```python
from build123d import *

# Parameters (mm, degrees)
SKETCH1_R           = 1.65
BOSS_EXTRUDE1_DEPTH = 30
SKETCH2_R           = 3
BOSS_EXTRUDE2_DEPTH = 3
FILLET1_R           = 5


with BuildPart() as part:
    # Sketch1 → Boss-Extrude1 (new body)
    with BuildSketch(Plane(origin=(0, 0, 0), x_dir=(1, 0, 0), z_dir=(0, 1, 0))):
        with Locations(Location((0, 0, 0), (0, 0, 270))):
            Circle(SKETCH1_R)
    extrude(amount=BOSS_EXTRUDE1_DEPTH)

    # Sketch2 → Boss-Extrude2 (add)
    with BuildSketch(Plane(origin=(0, 30, 0), x_dir=(1, 0, 0), z_dir=(0, 1, 0))):
        with Locations(Location((0, 0, 0), (0, 0, 270))):
            Circle(SKETCH2_R)
    extrude(amount=BOSS_EXTRUDE2_DEPTH)

    # Fillet1
    # the kernel refuses this fillet: 5 mm, written as the material it adds along each edge
    with BuildSketch(Plane(origin=(0, 30, 0), x_dir=(0, 0, 1), z_dir=(-1, 0, 0))) as fillet1_piece_1:
        with BuildLine():
            CenterArc((6.65, -3.417235725), FILLET1_R, 136.886394054, 43.113605946)
            Line((1.65, -3.417235725), (1.55, -3.417235725))
            Line((1.55, -3.417235725), (1.55, 0))
            Line((1.55, 0), (1.65, 0.1))
            ThreePointArc((1.65, 0.1), (2.325, 0.1), (2.927, 0.068344714))
            Line((2.927, 0.068344714), (3, 0))
        make_face()
    revolve(axis=Axis((0, 30, 0), (0, 1, 0)))


solid = part.part
```
Model file for the job. Use its own axes, mm. A direction names the side the tool comes from. Give positions to 0.01 mm unless a question says otherwise; leave off trailing zeros. Write each loop counter-clockwise with the first axis right and the second up, starting at its lowest first coordinate (ties: lowest second). Pieces come first, ordered by that corner, then holes. Notation, with made-up numbers: M -12,-11 L 5,-11 A16 ccw 5,10 Z; hole C 84.25,70.25 d3. An arc over 180 degrees is marked long. Use a Markdown table: item, result.
1) Pin check, flat tips, straight feed: pin 1 (3 mm diameter, centred on x = -0.5, y = 25, fed in from +Z); pin 2 (2 mm diameter, centred on y = 22.5, z = 1.5, fed in from +X); pin 3 (3 mm diameter, centred on y = 14, z = -2, fed in from -X). Stop position of each tip, or through.
Responses:
| item | result |
|---|---|
| pin 1 | stops at z = 1.65 |
| pin 2 | stops at x = 1.57 |
| pin 3 | stops at x = -1.57 |
2) Cut at B-B (z = 0). List the corners of the cut face in (x, y).
Responses:
| item | result |
|---|---|
| outline | M -3,30 A5 cw -1.65,26.58 L -1.65,0 L 1.65,0 L 1.65,26.58 A5 cw 3,30 L 3,33 L -3,33 Z |
3) Cut at A-A (x = 0). List the corners of the cut face in (y, z).
Responses:
| item | result |
|---|---|
| outline | M 0,-1.65 L 26.58,-1.65 A5 cw 30,-3 L 33,-3 L 33,3 L 30,3 A5 cw 26.58,1.65 L 0,1.65 Z |
4) Drill centre lines: line 1 (X direction, y = 6, z = 0); line 2 (Y direction, x = -0.4, z = 2.5); line 3 (X direction, y = 16.5, z = 1.5). Where is each one in solid material? Low to high. Write a range as from..to.
Responses:
| item | result |
|---|---|
| line 1 | x = -1.65..1.65 |
| line 2 | y = 29.42..33 |
| line 3 | x = -0.69..0.69 |
5) Cut at C-C (y = 8). List the corners of the cut face in (x, z), and give its area (3 significant figures).
Responses:
| item | result |
|---|---|
| outline | C 0,0 d3.3 |
| area | 8.55 mm2 |
6) Tool access for faces 1 (the cylindrical face through (-1, 13.11, -1.31)), 2 (the cylindrical face through (0.9, 31.48, 2.86)): list every direction of +Z, -Z, +X, -X, +Y, -Y with a clear straight run to the whole face (end or side of a thin tool).
Responses:
| item | result |
|---|---|
| face 1 | -Y |
| face 2 | +Y, -Y |
